For this review, use the dimensioned drawing (mm, ordinates from the lowest corner) and the shaded views. Coordinates: 2 decimals unless noted, no trailing zeros. Loops run counter-clockwise (first coordinate to the right, second up) from the corner with the lowest first, then second, coordinate; pieces in that order, holes last. Notation, with made-up numbers: (35, 57.25) - (50, 57.25) arc R30 ccw to (50, 95.25) - close; hole circle Ø7 at (-34.75, -6.75). An arc over 180 degrees is marked (long way). Answer in a Markdown table with one row per item. Add a question column.
(1) Mouldability with a two-part tool opening along Z and no side actions: class the marked faces 1, 2, 3 and 4 as +Z half, -Z half, draft (parallel to the pull), parting line (faces both ways), or undercut.
(2) We need section C-C on x = 23.5. Write out the cut boundary in (y, z).
(3) For line 1 along Z through (x, y) = (46, 11.25); line 2 along X through (y, z) = (3.25, 75); line 3 along Z through (x, y) = (32.5, 0.5), list the stretches that pass through material, from the lowest coordinate up.
(4) We need section A-A on z = 46. Write out the cut boundary in (x, y), plus the area to 3 significant figures.
(5) For P1, Ø6, axis at x = 82, z = 60.5, coming from the -Y side; P2, Ø5, axis at x = 49.5, y = 7, coming from the -Z side, all flat-tipped, find the tip position at first contact; note any pin that passes through.
(6) We need section B-B on y = 5.75. Write out the cut boundary in (x, z) (3 decimals), plus the area to 3 significant figures.
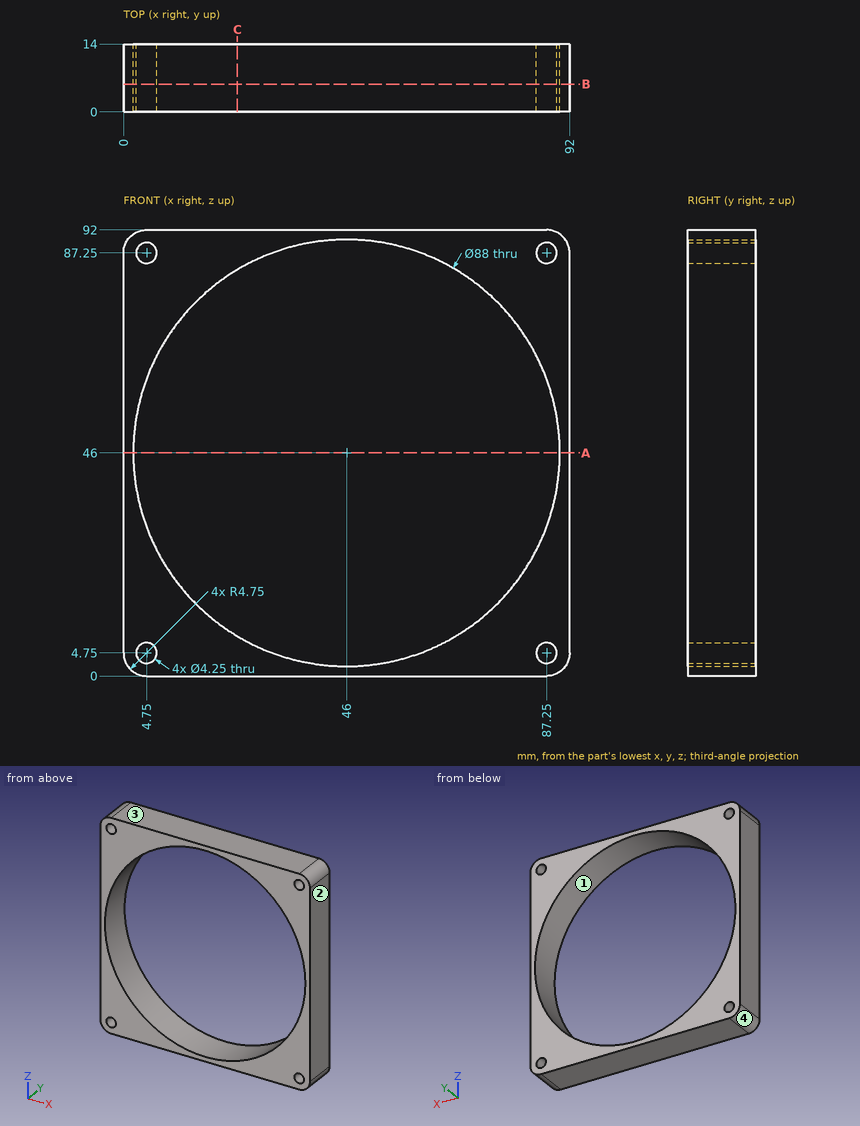
Outcome:
| question | item | result |
|---|---|---|
| 1 | face 1 | undercut |
| 1 | face 2 | draft |
| 1 | face 3 | +Z half |
| 1 | face 4 | -Z half |
| 2 | outline | (0, 0) - (14, 0) - (14, 8.19) - (0, 8.19) - close; (0, 83.81) - (14, 83.81) - (14, 92) - (0, 92) - close |
| 3 | line 1 | 0 to 2, 90 to 92 |
| 3 | line 2 | 0 to 12.91, 79.09 to 92 |
| 3 | line 3 | 0 to 4.12, 87.88 to 92 |
| 4 | outline | (0, 0) - (2, 0) - (2, 14) - (0, 14) - close; (90, 0) - (92, 0) - (92, 14) - (90, 14) - close |
| 4 | area | 56.0 mm² |
| 5 | P1 | through |
| 5 | P2 | z = 0 |
| 6 | outline | (0, 4.75) arc R4.75 ccw to (4.75, 0) - (87.25, 0) arc R4.75 ccw to (92, 4.75) - (92, 87.25) arc R4.75 ccw to (87.25, 92) - (4.75, 92) arc R4.75 ccw to (0, 87.25) - close; hole circle Ø88 at (46, 46); hole circle Ø4.25 at (4.75, 4.75); hole circle Ø4.25 at (4.75, 87.25); hole circle Ø4.25 at (87.25, 4.75); hole circle Ø4.25 at (87.25, 87.25) |
| 6 | area | 2,310 mm² |
